Geometry: see drawing. Coordinates: mm, zero at the bounding-box minimum. A direction names the side the tool comes from. Coordinates: 2 decimals unless noted, no trailing zeros. Write each loop counter-clockwise with the first axis right and the second up, starting at its lowest first coordinate (ties: lowest second). Pieces come first, ordered by that corner, then holes.
1) Section query A-A (z = 29). Output: boundary loops of the cut face in (x, y), then the cut area to 4 significant figures.
2) Section query C-C (y = 36.5). Output: boundary loops of the cut face in (x, z).
3) Pin query (flat end, axial travel): pin 1 Ø3 at (x, z) = (44.5, 32.5) entering from +Y; pin 2 Ø1.5 at (x, z) = (33, 29.5) entering from +Y; pin 3 Ø8 at (x, y) = (44.5, 24.5) entering from +Z. Return the tip coordinate at first contact, or that it passes through.
4) Section query B-B (x = 46). Output: boundary loops of the cut face in (y, z), then the cut area to 3 significant figures.
5) Section query D-D (x = 22). Output: boundary loops of the cut face in (y, z).
6) Line query: L1, parallel to Z at x = 36, y = 33.5; L2, parallel to Y at x = 46.5, z = 17. Output: solid intervals per line, ascending.
7) Set-up query: the marked faces 1 and 2. Return all of +Z, -Z, +X, -X, +Y, -Y with unobstructed straight access to the full face (end or side cutting, diameter ignored); none if empty.
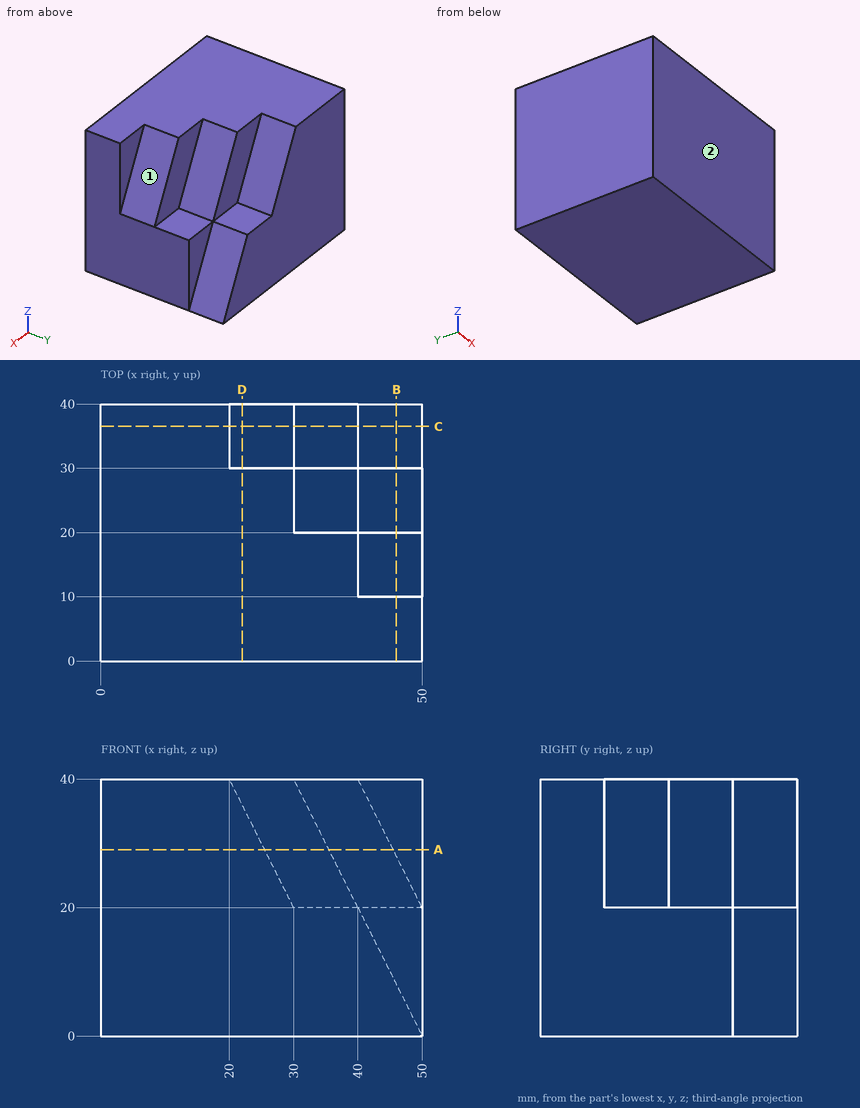
Answer:
1. outline: (0, 0) - (50, 0) - (50, 10) - (45.5, 10) - (45.5, 20) - (35.5, 20) - (35.5, 30) - (25.5, 30) - (25.5, 40) - (0, 40) - close
1. area: 1,565 mm2
2. outline: (0, 0) - (50, 0) - (40, 20) - (30, 20) - (20, 40) - (0, 40) - close
3. pin 1: stops at y = 20
3. pin 2: stops at y = 30
3. pin 3: stops at z = 20
4. outline: (0, 0) - (40, 0) - (40, 8) - (30, 8) - (30, 20) - (20, 20) - (20, 28) - (10, 28) - (10, 40) - (0, 40) - close
4. area: 960 mm2
5. outline: (0, 0) - (40, 0) - (40, 36) - (30, 36) - (30, 40) - (0, 40) - close
6. L1: z = 0 to 20
6. L2: y = 0 to 30
7. face 1: +Z, +X, +Y
7. face 2: +Z, -Z, +X, -X, -Y
